Geometry: see drawing. Coordinates: mm, zero at the bounding-box minimum. A direction names the side the tool comes from. Coordinates: 2 decimals unless noted, no trailing zeros. Write each loop counter-clockwise with the first axis right and the second up, starting at its lowest first coordinate (ties: lowest second). Pieces come first, ordered by that corner, then holes. Notation, with made-up numbers: (-5, 47.25) - (46, 47.25) arc R21 cw to (46, 56.25) - close; hole circle Ø5 at (34.5, 52). An arc over 180 degrees is marked (long way). One line per question, with ' | ' between items. Start each with the question number.
Q1. Line query: line 1 (X direction, y = 63, z = 4); line 2 (Y direction, x = 77, z = 63); line 3 (Z direction, x = 70, y = 38.1). Output: solid intervals per line, ascending.
Q2. Cut plane B-B, the plane z = 63.5. Return loops of the section in (x, y), plus the area to 3 significant figures.
Q3. Access query for the marked faces 4, 5 and 6. Directions: +Z, -Z, +X, -X, +Y, -Y. A direction counts if a zero-diameter tool reaches every point of the face in a straight line with its end or side. Return the directions, or none.
Q4. Cut plane C-C, the plane x = 28.5. Return loops of the section in (y, z).
Q5. Cut plane A-A, the plane y = 38.1. Return loops of the section in (x, z).
Q6. Draft query along Z for the marked faces 1, 2 and 3. Return one class per face: +Z half, -Z half, draft (parallel to the pull), parting line (faces both ways), or undercut.
Q7. Contact query for flat-ended pins moving along their axis: P1, Ø4, axis at y = 10, z = 3.5, coming from the -X side; P2, Ø4, axis at x = 15, z = 8.5, coming from the -Y side; P3, Ø7.5, axis at x = 97.5, z = 56.5, coming from the -Y side. Output: stop coordinate, or through.
Q8. Cut plane D-D, the plane z = 6.5. Return loops of the section in (x, y), plus the area to 3 significant figures.
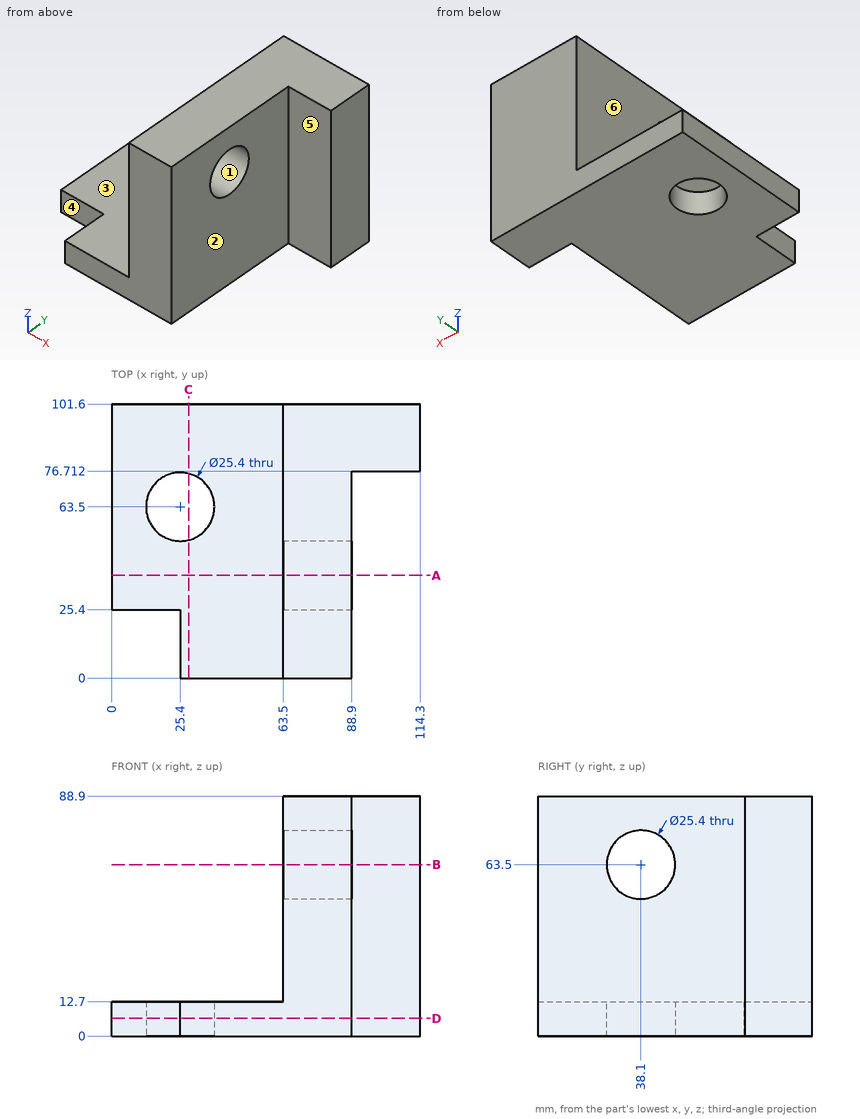
Reply:
1) line 1: x = 0 to 12.71, 38.09 to 88.9 | line 2: y = 0 to 25.41, 50.79 to 101.6 | line 3: z = 0 to 50.8, 76.2 to 88.9
2) outline: (63.5, 0) - (88.9, 0) - (88.9, 25.4) - (63.5, 25.4) - close; (63.5, 50.8) - (88.9, 50.8) - (88.9, 76.71) - (114.3, 76.71) - (114.3, 101.6) - (63.5, 101.6) - close | area: 2,570 mm^2
3) face 4: +Z, -Z, -X, -Y | face 5: +Z, -Z, +X, -Y | face 6: +Z, -X, +Y, -Y
4) outline: (0, 0) - (51.18, 0) - (51.18, 12.7) - (0, 12.7) - close; (75.82, 0) - (101.6, 0) - (101.6, 12.7) - (75.82, 12.7) - close
5) outline: (0, 0) - (88.9, 0) - (88.9, 50.8) - (63.5, 50.8) - (63.5, 12.7) - (0, 12.7) - close; (63.5, 76.2) - (88.9, 76.2) - (88.9, 88.9) - (63.5, 88.9) - close
6) face 1: undercut | face 2: draft | face 3: +Z half
7) P1: stops at x = 25.4 | P2: stops at y = 25.4 | P3: stops at y = 76.71
8) outline: (0, 25.4) - (25.4, 25.4) - (25.4, 0) - (88.9, 0) - (88.9, 76.71) - (114.3, 76.71) - (114.3, 101.6) - (0, 101.6) - close; hole circle Ø25.4 at (25.4, 63.5) | area: 8,510 mm^2
